Verification items for the finished model (mm, model axes). A direction names the side the tool comes from. Round coordinates to 2 decimals unless told otherwise and drop trailing zeros. Write each loop counter-clockwise with the first axis right and the second up, starting at its lowest first coordinate (ties: lowest second). Pieces come first, ordered by that corner, then holes. Notation, with made-up numbers: M 25.25,76.25 L 29.25,76.25 A24 ccw 29.25,87.25 Z; hole C -21.5,-17 d2. An arc over 180 degrees is marked long. Write each question's results on one line, items separated by ' | '.
from build123d import *

# Parameters (mm, degrees)
IZIM1_R                     = 4.8
Y_KSEKLIK_EKSTR_ZYON1_DEPTH = 10
IZIM2_R                     = 2.5
KES_EKSTR_ZYON1_DEPTH       = 7
IZIM3_R                     = 1
KES_EKSTR_ZYON2_DEPTH       = 5.8
IZIM4_W                     = 1.6
IZIM4_H                     = 4
KES_EKSTR_ZYON3_DEPTH       = 5


with BuildPart() as part:
    # Çizim1 → Yükseklik-Ekstrüzyon1 (new body)
    with BuildSketch(Plane(origin=(0, 0, 0), x_dir=(1, 0, 0), z_dir=(0, 1, 0))):
        Circle(IZIM1_R)
    extrude(amount=Y_KSEKLIK_EKSTR_ZYON1_DEPTH)

    # Çizim2 → Kes-Ekstrüzyon1 (cut)
    with BuildSketch(Plane(origin=(0, 10, 0), x_dir=(1, 0, 0), z_dir=(0, 1, 0))):
        Circle(IZIM2_R)
    extrude(amount=-KES_EKSTR_ZYON1_DEPTH, mode=Mode.SUBTRACT)

    # Çizim3 → Kes-Ekstrüzyon2 (cut, through all)
    with BuildSketch(Plane(origin=(0, 0, 0), x_dir=(0, 0, -1), z_dir=(1, 0, 0))):
        with Locations((0, 7)):
            Circle(IZIM3_R)
    extrude(amount=-KES_EKSTR_ZYON2_DEPTH, mode=Mode.SUBTRACT)

    # Çizim4 → Kes-Ekstrüzyon3 (cut)
    with BuildSketch(Plane(origin=(0, 10, 0), x_dir=(1, 0, 0), z_dir=(0, 1, 0))):
        with Locations((-3.45, 0)):
            Rectangle(IZIM4_W, IZIM4_H)
    extrude(amount=-KES_EKSTR_ZYON3_DEPTH, mode=Mode.SUBTRACT)


solid = part.part
1) Depth check by flat-ended pin: P1, Ø1.2, axis at y = 7.5, z = -1, coming from the +X side; P2, Ø0.8, axis at x = -3, y = 8.5, coming from the +Z side; P3, Ø1.8, axis at x = -3.5, z = -0.5, coming from the +Y side; P4, Ø1.6, axis at y = 7, z = 0, coming from the -X side. Enter the tip coordinate at first touch or a pass-through.
Calculated:
P1: stops at x = 4.78 | P2: stops at z = 4.03 | P3: stops at y = 10 | P4: stops at x = 2.37
2) Sectioned sample at D-D, the plane z = -1.5. Record the cut outline in (x, y).
Calculated:
outline: M -4.56,0 L 4.56,0 L 4.56,10 L 2,10 L 2,3 L -2,3 L -2,10 L -2.65,10 L -2.65,5 L -4.25,5 L -4.25,10 L -4.56,10 Z
3) Draft check along X on faces 1 (the flat face through (0, 0, 0)), 2 (the flat face through (-3, 5, 0)), 3 (the cylindrical face through (4.58, 4.93, -1.44)). Enter one of: pulls with the +X half, pulls with the -X half, needs draft (parallel to the pull), parting line crosses it, or undercut.
Calculated:
face 1: needs draft | face 2: undercut | face 3: parting line crosses it
4) Sectioned sample at C-C, the plane y = 3.75. Record the cut outline in (x, z), and give its area (3 significant figures).
Calculated:
outline: C 0,0 d9.6; hole C 0,0 d5 | area: 52.7 mm²
5) Sectioned sample at A-A, the plane z = 0. Record the cut outline in (x, y), and give its area (3 significant figures).
Calculated:
outline: M -4.8,0 L 4.8,0 L 4.8,10 L 2.5,10 L 2.5,3 L -2.5,3 L -2.5,6 L -2.65,6 L -2.65,5 L -4.25,5 L -4.25,6 L -4.8,6 Z; M -4.8,8 L -4.25,8 L -4.25,10 L -4.8,10 Z; M -2.65,8 L -2.5,8 L -2.5,10 L -2.65,10 Z | area: 51.6 mm²
6) Sectioned sample at B-B, the plane x = 0. Record the cut outline in (y, z).
Calculated:
outline: M 0,-4.8 L 10,-4.8 L 10,-2.5 L 3,-2.5 L 3,2.5 L 10,2.5 L 10,4.8 L 0,4.8 Z
7) Access from +Z, -Z, +X, -X, +Y, -Y to the whole of each face (thin tool, end or side, straight path). Record for faces 4 (the flat face through (-2.65, 8.1, 0.5)), 5 (the cylindrical face through (-4.522, 6.617, -0.924)), 6 (the flat face through (2, 10, 2)).
Calculated:
face 4: +Y | face 5: -X | face 6: +Z, -Z, +X, -X, +Y
8) Material ranges on line 1 (Y direction, x = -4.6, z = 0); line 2 (X direction, y = 9.5, z = 0.5); line 3 (X direction, y = 9.75, z = 0.25), recorded low to high. Write a range as [from, to].
Calculated:
line 1: y = [0, 6], [8, 10] | line 2: x = [-4.77, -4.25], [-2.65, -2.45], [2.45, 4.77] | line 3: x = [-4.79, -4.25], [-2.65, -2.49], [2.49, 4.79]
